from build123d import *

# Parameters (mm, degrees)
F0_R     = 10
F1_DEPTH = 30
F2_R     = 2.5
F3_DEPTH = 5.001


with BuildPart() as f1:
    # F0 (on Front) → F1 (new body, symmetric)
    with BuildSketch(Plane.XZ):
        with BuildLine():
            Line((-60, -81.240696), (-100, -81.240696))
            Line((-100, -81.240696), (-100, -86.240696))
            Line((-100, -86.240696), (-56.557951, -86.240696))
            Line((-56.557951, -86.240696), (-39.363156, -41.240696))
            Line((-39.363156, -41.240696), (-37.452623, -36.240696))
            Line((-37.452623, -36.240696), (-13.331959, 26.884796))
            ThreePointArc((-13.331959, 26.884796), (-14.976864, 32.926515), (-14.011929, 39.113354))
            Line((-14.011929, 39.113354), (-60, -81.240696))
        make_face()
        with BuildLine():
            Line((60, -81.240696), (14.011929, 39.113354))
            ThreePointArc((14.011929, 39.113354), (14.750914, 36.481534), (15, 33.759304))
            ThreePointArc((15, 33.759304), (14.577026, 30.222313), (13.331959, 26.884796))
            Line((13.331959, 26.884796), (37.452623, -36.240696))
            Line((37.452623, -36.240696), (39.363156, -41.240696))
            Line((39.363156, -41.240696), (56.557951, -86.240696))
            Line((56.557951, -86.240696), (100, -86.240696))
            Line((100, -86.240696), (100, -81.240696))
            Line((100, -81.240696), (60, -81.240696))
        make_face()
        with BuildLine():
            ThreePointArc((14.011929, 39.113354), (0, 48.759304), (-14.011929, 39.113354))
            ThreePointArc((-14.011929, 39.113354), (-14.976864, 32.926515), (-13.331959, 26.884796))
            ThreePointArc((-13.331959, 26.884796), (0, 18.759304), (13.331959, 26.884796))
            ThreePointArc((13.331959, 26.884796), (14.577026, 30.222313), (15, 33.759304))
            ThreePointArc((15, 33.759304), (14.750914, 36.481534), (14.011929, 39.113354))
        make_face()
        with Locations((0, 33.759304)):
            Circle(F0_R, mode=Mode.SUBTRACT)
        Polygon((-37.452623, -36.240696), (-39.363156, -41.240696), (39.363156, -41.240696), (37.452623, -36.240696), align=None)
    extrude(amount=F1_DEPTH, both=True)

    # F2 (on face) → F3 (cut, through all)
    with BuildSketch(Plane.XY.offset(-81.240696)):
        with Locations((-85, 15)):
            Circle(F2_R)
        with Locations((-85, -15)):
            Circle(F2_R)
        with Locations((85, -15)):
            Circle(F2_R)
        with Locations((85, 15)):
            Circle(F2_R)
    extrude(amount=-F3_DEPTH, mode=Mode.SUBTRACT)


solid = f1.part
Geometry check sheet. Reference: the model listing, model coordinates, mm. A direction names the side the tool comes from. Round coordinates to 2 decimals unless told otherwise and drop trailing zeros. Loops run counter-clockwise (first coordinate to the right, second up) from the corner with the lowest first, then second, coordinate; pieces in that order, holes last. Notation, with made-up numbers: (72.25, 2.25) -> (86.25, 2.25) arc R32 ccw to (86.25, 41.25) -> close; hole circle Ø7 at (14, 5.25). An arc over 180 degrees is marked (long way). Answer as a JSON object with one key per item and string values. Group by question number.
Item 1: Depth check by flat-ended pin: pin 1 Ø8 at (x, y) = (24.5, -22.5) entering from -Z; pin 2 Ø6 at (x, y) = (-85, 15) entering from +Z; pin 3 Ø2 at (y, z) = (8.5, -7.5) entering from +X. Enter the tip coordinate at first touch or a pass-through.
Item 2: Thickness scan on line 1 along Y through (x, z) = (85, -84.4); line 2 along Z through (x, y) = (8.5, 23); line 3 along Z through (x, y) = (-5.5, 5.5). Record the ranges inside material, lowest first.
Item 3: Cross-section at D-D, the plane x = -8. Record the cut outline in (y, z).
Item 4: Cross-section at B-B, the plane x = 85. Record the cut outline in (y, z), plus the area to 3 significant figures.
Item 5: Set-up check for faces 1 (the face through (80, 0, -81.241)), 2 (the face through (25.223, -0.42, -4.236)), 3 (the face through (-48.081, -0.42, -64.056)), 4 (the face through (78, 0, -86.241)): record each of +Z, -Z, +X, -X, +Y, -Y from which the full face is reachable in a straight line by a thin tool's end or side.
Item 6: Cross-section at A-A, the plane y = 15. Record the cut outline in (x, z), plus the area to 3 significant figures.
Item 7: Cross-section at C-C, the plane z = -57. Record the cut outline in (x, y).
Item 8: Release check for a two-part mould opening along Y. For faces 5 (the face through (0, -30, -38)), 6 (the face through (37.33, -0.42, -21.91)), 7 (the face through (-87, -16.5, -83.7)) record: pulls with the +Y half, pulls with the -Y half, needs draft (parallel to the pull), parting line crosses it, or undercut.
Determined:
{
 "1": {"pin 1": "stops at z = -41.24", "pin 2": "stops at z = -81.24", "pin 3": "stops at x = 32.21"},
 "2": {"line 1": "y = -30 to -17.5, -12.5 to 12.5, 17.5 to 30", "line 2": "z = -41.24 to -36.24, 21.4 to 28.49, 39.03 to 46.12", "line 3": "z = -41.24 to -36.24, 19.8 to 25.41, 42.11 to 47.71"},
 "3": {"outline": "(-30, -41.24) -> (30, -41.24) -> (30, -36.24) -> (-30, -36.24) -> close; (-30, 21.07) -> (30, 21.07) -> (30, 27.76) -> (-30, 27.76) -> close; (-30, 39.76) -> (30, 39.76) -> (30, 46.45) -> (-30, 46.45) -> close"},
 "4": {"outline": "(-30, -86.24) -> (-17.5, -86.24) -> (-17.5, -81.24) -> (-30, -81.24) -> close; (-12.5, -86.24) -> (12.5, -86.24) -> (12.5, -81.24) -> (-12.5, -81.24) -> close; (17.5, -86.24) -> (30, -86.24) -> (30, -81.24) -> (17.5, -81.24) -> close", "area": "250 mm²"},
 "5": {"face 1": "+Z, +X, +Y, -Y", "face 2": "+Y, -Y", "face 3": "-Z, +Y, -Y", "face 4": "-Z, +X, -X, +Y, -Y"},
 "6": {"outline": "(-100, -86.24) -> (-87.5, -86.24) -> (-87.5, -81.24) -> (-100, -81.24) -> close; (-82.5, -86.24) -> (-56.56, -86.24) -> (-39.36, -41.24) -> (39.36, -41.24) -> (56.56, -86.24) -> (82.5, -86.24) -> (82.5, -81.24) -> (60, -81.24) -> (14.01, 39.11) arc R15 ccw to (-14.01, 39.11) -> (-60, -81.24) -> (-82.5, -81.24) -> close; (87.5, -86.24) -> (100, -86.24) -> (100, -81.24) -> (87.5, -81.24) -> close; hole (-37.45, -36.24) -> (37.45, -36.24) -> (13.33, 26.88) arc R15 cw to (-13.33, 26.88) -> close; hole circle Ø20 at (0, 33.76)", "area": "2,370 mm²"},
 "7": {"outline": "(-50.74, -30) -> (-45.38, -30) -> (-45.38, 30) -> (-50.74, 30) -> close; (45.38, -30) -> (50.74, -30) -> (50.74, 30) -> (45.38, 30) -> close"},
 "8": {"face 5": "pulls with the -Y half", "face 6": "needs draft", "face 7": "undercut"}
}
